```python
from build123d import *

# Parameters (mm, degrees)
BOSS_EXTRUDE1_DEPTH = 6
SKETCH2_R           = 1.5
BOSS_EXTRUDE2_DEPTH = 6
SKETCH3_R           = 1.5
CUT_EXTRUDE1_DEPTH  = 4


with BuildPart() as part:
    # Sketch1 → Boss-Extrude1 (new body)
    with BuildSketch(Plane(origin=(0, 0, 0), x_dir=(1, 0, 0), z_dir=(0, 1, 0))):
        Polygon((0, -3.233161507), (2.8, -1.616580754), (2.8, 1.616580754), (0, 3.233161507), (-2.8, 1.616580754), (-2.8, -1.616580754), align=None)
    extrude(amount=BOSS_EXTRUDE1_DEPTH)

    # Sketch2 → Boss-Extrude2 (add)
    with BuildSketch(Plane(origin=(0, 0, 0), x_dir=(-1, 0, 0), z_dir=(0, -1, 0))):
        Circle(SKETCH2_R)
    extrude(amount=BOSS_EXTRUDE2_DEPTH)

    # Sketch3 → Cut-Extrude1 (cut)
    with BuildSketch(Plane(origin=(0, 6, 0), x_dir=(1, 0, 0), z_dir=(0, 1, 0))):
        Circle(SKETCH3_R)
    extrude(amount=-CUT_EXTRUDE1_DEPTH, mode=Mode.SUBTRACT)


solid = part.part
```
CAD build for the part. Positions are in the model's coordinates, mm. A direction names the side the tool comes from. Coordinates: 2 decimals unless noted, no trailing zeros. Write each loop counter-clockwise with the first axis right and the second up, starting at its lowest first coordinate (ties: lowest second). Pieces come first, ordered by that corner, then holes.
(1) Two-plate mould, pull along Z, no slides. Class faces 1 (the face through (-1.42, 2.958, 2.414)), 2 (the face through (-1.3, 0, 1.4)), 3 (the face through (0, 2, 0)): +Z half, -Z half, draft (parallel to the pull), parting line (faces both ways), or undercut.
(2) Drill centre lines: probe 1 along X at (y, z) = (4, 0); probe 2 along Y at (x, z) = (-1, -0.5); probe 3 along X at (y, z) = (3.75, 0.75). Where is each one in solid material? Low to high.
(3) 3-axis set-ups, long thin cutter, end or side, ignore diameter. For faces 4 (the face through (-1.5, 4.03, -0.07)), 5 (the face through (1.5, -2.96, -0.07)), 6 (the face through (-2.8, 3, 0)): which of +Z, -Z, +X, -X, +Y, -Y reach the whole face in a straight line?
(4) Cut at C-C, the plane x = -0.85. List the corners of the cut face in (y, z), and give its area (3 significant figures).
(5) Cut at A-A, the plane y = 2.75. List the corners of the cut face in (x, z), and give its area (3 significant figures).
(6) Flat gauge pins, fed straight in: pin 1 (1 mm diameter, centred on x = 1, y = -4.5, fed in from +Z); pin 2 (2 mm diameter, centred on x = -0.5, y = 4.5, fed in from -Z). Where does each tip first touch, or does it go through?
(7) Cut at D-D, the plane y = 0.25. List the corners of the cut face in (x, z).
(8) Cut at B-B, the plane z = 0. List the corners of the cut face in (x, y), and give its area (3 significant figures).
Geometry says:
1. face 1: +Z half
1. face 2: draft
1. face 3: undercut
2. probe 1: x = -2.8 to -1.5, 1.5 to 2.8
2. probe 2: y = -6 to 2
2. probe 3: x = -2.8 to -1.3, 1.3 to 2.8
3. face 4: +Y
3. face 5: -Y
3. face 6: +Z, -Z, -X, +Y, -Y
4. outline: (-6, -1.24) - (0, -1.24) - (0, -2.74) - (6, -2.74) - (6, -1.24) - (2, -1.24) - (2, 1.24) - (6, 1.24) - (6, 2.74) - (0, 2.74) - (0, 1.24) - (-6, 1.24) - close
4. area: 37.9 mm2
5. outline: (-2.8, -1.62) - (0, -3.23) - (2.8, -1.62) - (2.8, 1.62) - (0, 3.23) - (-2.8, 1.62) - close; hole circle Ø3 at (0, 0)
5. area: 20.1 mm2
6. pin 1: stops at z = 1.41
6. pin 2: stops at z = -3.23
7. outline: (-2.8, -1.62) - (0, -3.23) - (2.8, -1.62) - (2.8, 1.62) - (0, 3.23) - (-2.8, 1.62) - close
8. outline: (-2.8, 0) - (-1.5, 0) - (-1.5, -6) - (1.5, -6) - (1.5, 0) - (2.8, 0) - (2.8, 6) - (1.5, 6) - (1.5, 2) - (-1.5, 2) - (-1.5, 6) - (-2.8, 6) - close
8. area: 39.6 mm2
